CAD build for the part. Positions are in the model's coordinates, mm. A direction names the side the tool comes from. Coordinates: 2 decimals unless noted, no trailing zeros. Write each loop counter-clockwise with the first axis right and the second up, starting at its lowest first coordinate (ties: lowest second). Pieces come first, ordered by that corner, then holes.
```python
from build123d import *

# Parameters (mm, degrees)
SKETCH_3_W             = 11.653142641
SKETCH_3_H             = 0.953639491
CUT_EXTRUDE_1_DEPTH    = 12
HOLE_WIZARD_M3_1_D     = 2.5
HOLE_WIZARD_M3_1_DEPTH = 7.5
HOLE_WIZARD_M3_1_TIP   = 0.751075774


with BuildPart() as part:
    # 草图1 → 旋转1 (revolve)
    with BuildSketch(Plane.XY):
        Polygon((0, 0), (46, 0), (46, 18.5), (23, 18.5), (23, 16.5), (0, 16.5), align=None)
    revolve(axis=Axis((0, 0, 0), (1, 0, 0)))

    # 草图2 → 旋转2 (revolve)
    with BuildSketch(Plane.XY):
        Polygon((46, 7), (64, 7), (64, 4), (52, 4), (52, 1), (46, 1), align=None)
    revolve(axis=Axis((46, 7, 0), (1, 0, 0)))

    # 草图3 → 切除-拉伸1 (cut)
    with BuildSketch(Plane(origin=(64, 0, 0), x_dir=(0, 0, -1), z_dir=(1, 0, 0))):
        with Locations((-0.372215264, 9.976819746)):
            Rectangle(SKETCH_3_W, SKETCH_3_H)
    extrude(amount=-CUT_EXTRUDE_1_DEPTH, mode=Mode.SUBTRACT)

    # M3 螺纹孔1
    with Locations(Plane(origin=(46, 0, 0), x_dir=(0, 0, -1), z_dir=(1, 0, 0))):
        with Locations((-7.75, 13.423393759), (7.75, 13.423393759), (15.4165108, 0.144607536), (7.75, -13.423393759), (-7.75, -13.423393759), (-15.5, 0)):
            Hole(HOLE_WIZARD_M3_1_D / 2, depth=HOLE_WIZARD_M3_1_DEPTH)
            with Locations((0, 0, -(HOLE_WIZARD_M3_1_DEPTH + HOLE_WIZARD_M3_1_TIP / 2))):  # 118° drill point
                Cone(0, HOLE_WIZARD_M3_1_D / 2, HOLE_WIZARD_M3_1_TIP, mode=Mode.SUBTRACT)


solid = part.part
```
Item 1: Which spindle directions (+Z, -Z, +X, -X, +Y, -Y) get a long thin tool onto all of the face, cutting with end or side? Do faces 1 (the flat face through (52, 10, 0)), 2 (the cylindrical face through (11.34, 15.24, -6.32)), 3 (the flat face through (0, 0, 0)). Say none if no direction does.
Item 2: Saw through at B-B, the plane y = -9. Write the cut outline in (x, z), and give its area (3 significant figures).
Item 3: Saw through at A-A, the plane x = 42. Write the cut outline in (y, z).
Item 4: Wall check: line 1 along Z through (x, y) = (42.75, 0); line 2 along X through (y, z) = (12, 14); line 3 along Y through (x, z) = (42, 7). Give the ranges that are in metal, low to high.
Item 5: Flat gauge pins, fed straight in: pin 1 Ø4 at (x, y) = (42, 13) entering from -Z; pin 2 Ø2.5 at (x, z) = (55, 0) entering from +Y; pin 3 Ø2 at (y, z) = (7, 8.5) entering from +X. Where does each tip first touch, or does it go through?
Item 6: Two-plate mould, pull along Y, no slides. Class faces 4 (the cylindrical face through (34.34, -4.01, -18.06)), 5 (the cylindrical face through (42.2, -12.58, -8.67)), 6 (the flat face through (64, 7, 0)): +Y half, -Y half, draft (parallel to the pull), parting line (faces both ways), or undercut.
Item 7: Saw through at D-D, the plane z = -4. Write the cut outline in (x, y), and give its area (3 significant figures).
Item 8: Saw through at C-C, the plane x = 6. Write the cut outline in (y, z).
Working result:
1. face 1: +X
1. face 2: -X
1. face 3: +Z, -Z, -X, +Y, -Y
2. outline: (0, -13.83) - (23, -13.83) - (23, -16.16) - (46, -16.16) - (46, 16.16) - (23, 16.16) - (23, 13.83) - (0, 13.83) - close
2. area: 1,380 mm2
3. outline: circle Ø37 at (0, 0); hole circle Ø2.5 at (-13.42, -7.75); hole circle Ø2.5 at (-13.42, 7.75); hole circle Ø2.5 at (0, 15.5); hole circle Ø2.5 at (0.14, -15.42); hole circle Ø2.5 at (13.42, -7.75); hole circle Ø2.5 at (13.42, 7.75)
4. line 1: z = -18.5 to -16.66, -14.17 to 14.25, 16.75 to 18.5
4. line 2: x = 23 to 46
4. line 3: y = -17.12 to -14.42, -12.42 to 12.42, 14.42 to 17.12
5. pin 1: stops at z = -14.87
5. pin 2: stops at y = 9.5
5. pin 3: stops at x = 46
6. face 4: parting line
6. face 5: undercut
6. face 6: draft
7. outline: (0, -16.01) - (23, -16.01) - (23, -18.06) - (46, -18.06) - (46, 2.53) - (52, 2.53) - (52, 11.47) - (46, 11.47) - (46, 18.06) - (23, 18.06) - (23, 16.01) - (0, 16.01) - close
7. area: 1,620 mm2
8. outline: circle Ø33 at (0, 0)
